The figure shows three views and two pictorial views of one solid part (mm, origin at its lowest corner). Answer the questions. A direction names the side the tool comes from. Coordinates: 2 decimals unless noted, no trailing zeros. Loops run counter-clockwise (first coordinate to the right, second up) from the corner with the lowest first, then second, coordinate; pieces in that order, holes last. Notation, with made-up numbers: (48.5, 71) - (62.5, 71) arc R15 ccw to (62.5, 86) - close; hole circle Ø10 at (63, 21). An arc over 180 degrees is marked (long way). Write each question's results on one line, items separated by ' | '. Start each with the question number.
Item 1: A tool of negligible diameter and unlimited length cuts with its end or side. For the marked faces 1 and 2, from which of +Z, -Z, +X, -X, +Y, -Y can it reach the whole face along a straight path? Write none if from no direction.
Item 2: Section C-C, the plane x = 47 is taken. Write down the section's boundary in (y, z), plus the area to 3 significant figures.
Item 3: Section D-D, the plane y = 5.5 is taken. Write down the section's boundary in (x, z).
Item 4: Each of these flat-tipped pins is pushed along its axis until it touches: pin 1 Ø1.5 at (y, z) = (32, 55.5) entering from -X; pin 2 Ø12 at (x, y) = (76.5, 32.5) entering from -Z; pin 3 Ø1.9 at (x, z) = (99, 13) entering from -Y. Where does it stop, or does it pass through?
Item 5: Consider probe 1 along X at (y, z) = (25.5, 63.5) (1 decimal); probe 2 along X at (y, z) = (33, 26); probe 3 along Z at (x, y) = (50, 10). Determine where each line is inside the solid, lowest interval first. Write a range as [from, to].
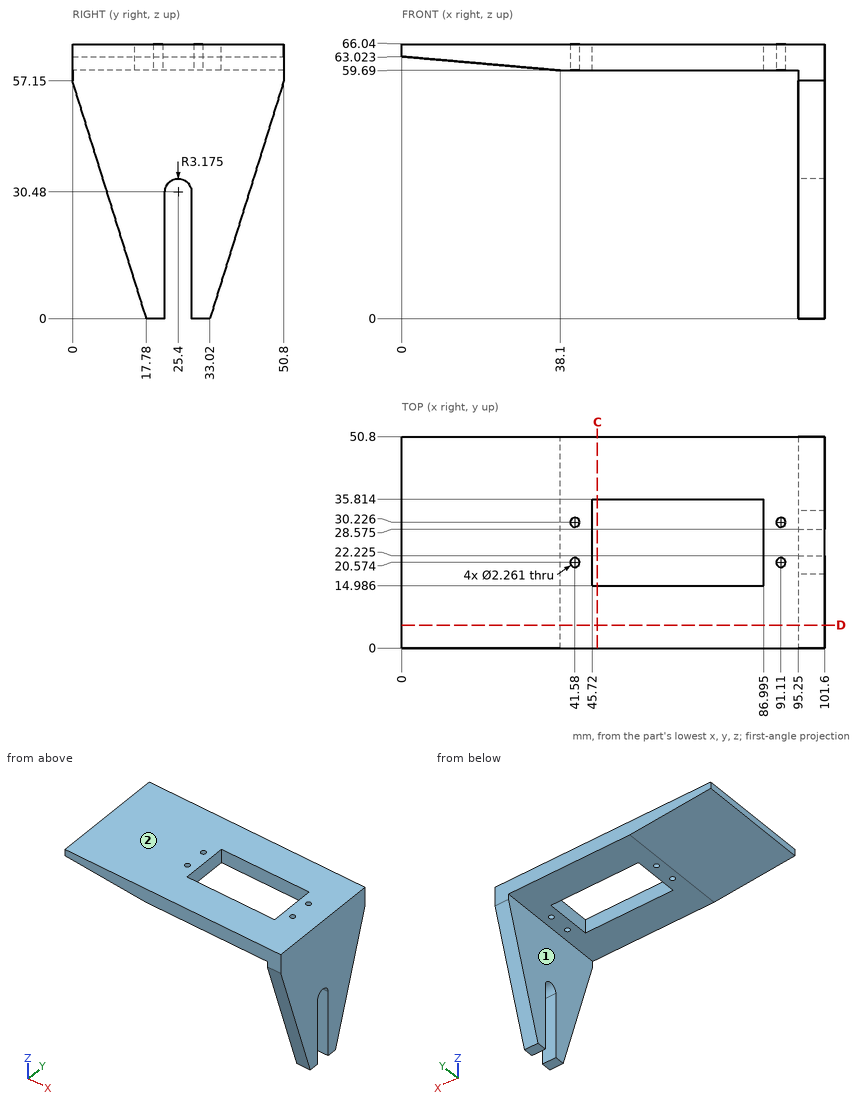
Answer key:
1) face 1: -Z, -X, +Y, -Y | face 2: +Z, +X, -X, +Y, -Y
2) outline: (0, 59.69) - (14.99, 59.69) - (14.99, 66.04) - (0, 66.04) - close; (35.81, 59.69) - (50.8, 59.69) - (50.8, 66.04) - (35.81, 66.04) - close | area: 190 mm^2
3) outline: (0, 63.02) - (38.1, 59.69) - (95.25, 59.69) - (95.25, 39.47) - (101.6, 39.47) - (101.6, 66.04) - (0, 66.04) - close
4) pin 1: stops at x = 95.25 | pin 2: stops at z = 59.69 | pin 3: stops at y = 13.44
5) probe 1: x = [0, 45.7], [87, 101.6] | probe 2: x = [95.25, 101.6] | probe 3: z = [59.69, 66.04]
